Design review of the part built by this model. Coordinates are the model's own, in mm. Face numbers are marked on the shaded views. A direction names the side the tool comes from. Give positions to 0.01 mm unless a question says otherwise; leave off trailing zeros. Order: outer loops, then holes, each group sorted by start corner. A loop starts at its lowest first (then second) coordinate and runs counter-clockwise, first axis right, second up. Notation, with made-up numbers: (88.25, -25.5) -> (98.25, -25.5) arc R32 ccw to (98.25, 4.5) -> close; hole circle Ø5 at (-12.5, -37). An arc over 180 degrees is marked (long way). One line per item, written item: value.
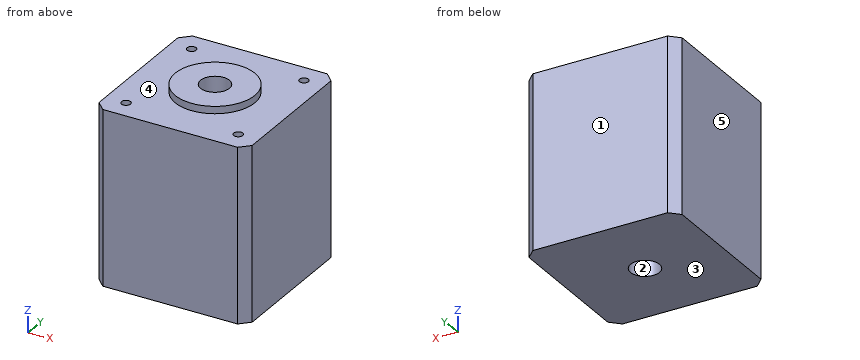
from build123d import *

# Parameters (mm, degrees)
SKETCH1_W                       = 42.3
SKETCH1_H                       = 42.3
BOSS_EXTRUDE1_DEPTH             = 48
TAP_DRILL_FOR_M3X0_5_TAP1_D     = 2.5
TAP_DRILL_FOR_M3X0_5_TAP1_DEPTH = 7.868
TAP_DRILL_FOR_M3X0_5_TAP1_TIP   = 0.751075774
SKETCH5_R                       = 11
BOSS_EXTRUDE2_DEPTH             = 2
SKETCH6_R                       = 4
CUT_EXTRUDE1_DEPTH              = 78.965248669
CHAMFER1_SIZE                   = 2.54


with BuildPart() as part:
    # Sketch1 → Boss-Extrude1 (new body)
    with BuildSketch(Plane.XY):
        with Locations((21.15, 21.15)):
            Rectangle(SKETCH1_W, SKETCH1_H)
    extrude(amount=BOSS_EXTRUDE1_DEPTH)

    # Tap Drill for M3x0.5 Tap1
    with Locations(Plane.XY.offset(48)):
        with Locations((36.65, 5.65), (36.65, 36.65), (5.65, 5.65), (5.65, 36.65)):
            Hole(TAP_DRILL_FOR_M3X0_5_TAP1_D / 2, depth=TAP_DRILL_FOR_M3X0_5_TAP1_DEPTH)
            with Locations((0, 0, -(TAP_DRILL_FOR_M3X0_5_TAP1_DEPTH + TAP_DRILL_FOR_M3X0_5_TAP1_TIP / 2))):  # 118° drill point
                Cone(0, TAP_DRILL_FOR_M3X0_5_TAP1_D / 2, TAP_DRILL_FOR_M3X0_5_TAP1_TIP, mode=Mode.SUBTRACT)

    # Sketch5 → Boss-Extrude2 (add)
    with BuildSketch(Plane.XY.offset(48)):
        with Locations(Location((21.15, 21.15, 0), (0, 0, 180))):
            Circle(SKETCH5_R)
    extrude(amount=BOSS_EXTRUDE2_DEPTH)

    # Sketch6 → Cut-Extrude1 (cut, through all)
    with BuildSketch(Plane.XY.offset(50)):
        with Locations((21.15, 21.15)):
            Circle(SKETCH6_R)
    extrude(amount=-CUT_EXTRUDE1_DEPTH, mode=Mode.SUBTRACT)

    # Chamfer1
    chamfer1_edges = [part.edges().sort_by_distance(p)[0] for p in [
        (0, 42.3, 24),
        (42.3, 42.3, 24),
        (42.3, 0, 24),
        (0, 0, 24),
    ]]
    chamfer(chamfer1_edges, length=CHAMFER1_SIZE)


solid = part.part
Item 1: Machinability: for the marked faces 4 and 5, which of the approach directions +Z, -Z, +X, -X, +Y, -Y give a long, thin tool a straight path to every point of the face, cutting with its end or side? Answer none if there is none.
Returned:
face 4: +Z
face 5: +Z, -Z, -X, +Y, -Y
Item 2: Draft analysis for pull direction Y (two halves, no side actions). For the marked faces 1, 2 and 3, state which applies: pulls with the +Y half, pulls with the -Y half, needs draft (parallel to the pull), parting line crosses it, or undercut.
Returned:
face 1: pulls with the +Y half
face 2: undercut
face 3: needs draft
Item 3: Add section D-D on y = 33. Give the boundary of the cut face in (x, z), plus the area to 3 significant figures.
Returned:
outline: (0, 0) -> (42.3, 0) -> (42.3, 48) -> (0, 48) -> close
area: 2,030 mm²
Item 4: Add section C-C on x = 31. Give the boundary of the cut face in (y, z).
Returned:
outline: (0, 0) -> (42.3, 0) -> (42.3, 48) -> (26.05, 48) -> (26.05, 50) -> (16.25, 50) -> (16.25, 48) -> (0, 48) -> close
Item 5: Add section B-B on y = 23. Give the boundary of the cut face in (x, z).
Returned:
outline: (0, 0) -> (17.6, 0) -> (17.6, 50) -> (10.31, 50) -> (10.31, 48) -> (0, 48) -> close; (24.7, 0) -> (42.3, 0) -> (42.3, 48) -> (31.99, 48) -> (31.99, 50) -> (24.7, 50) -> close
Item 6: Clearance check with flat-ended pins moving along their axes: P1, Ø6.5, axis at x = 21.15, y = 21.15, coming from the -Z side; P2, Ø2, axis at x = 36.65, y = 5.65, coming from the +Z side; P3, Ø3, axis at x = 5.65, y = 36.65, coming from the +Z side. State where each tip first meets the part, or that it passes through.
Returned:
P1: through
P2: z = 39.98
P3: z = 48
Item 7: Add section A-A on z = 5. Give the boundary of the cut face in (x, y), plus the area to 3 significant figures.
Returned:
outline: (0, 2.54) -> (2.54, 0) -> (39.76, 0) -> (42.3, 2.54) -> (42.3, 39.76) -> (39.76, 42.3) -> (2.54, 42.3) -> (0, 39.76) -> close; hole circle Ø8 at (21.15, 21.15)
area: 1,730 mm²
Item 8: To check wall thickness, follow line 1 along X through (y, z) = (36.65, 44); line 2 along X through (y, z) = (5, 45). State the ranges of each line that lie inside material, in increasing order. Write a range as from..to.
Returned:
line 1: 0..4.4, 6.9..35.4, 37.9..42.3
line 2: 0..4.58, 6.72..35.58, 37.72..42.3
